from build123d import *

# Parameters (mm, degrees)
BOSS_EXTRUDE1_DEPTH = 10
FILLET1_R           = 0.2
BOSS_EXTRUDE2_START = -0.1
SKETCH2_W           = 1.752559166
SKETCH2_H           = 10
BOSS_EXTRUDE2_DEPTH = 0.6
LPATTERN1_DEPTH     = 10


# Read off the part's stored shape, not the designer's step: LPattern1
with BuildPart() as part:
    # Sketch1 → Boss-Extrude1 (new body)
    with BuildSketch(Plane(origin=(0, 0, 0), x_dir=(1, 0, 0), z_dir=(0, 1, 0))):
        with BuildLine():
            Line((0, 3), (0, 0))
            Line((0, 0), (5, 0))
            Line((5, 0), (5, 3))
            Line((5, 3), (2.982182538, 3))
            ThreePointArc((2.982182538, 3), (3.252447725, 2.695376303), (3.35, 2.3))
            ThreePointArc((3.35, 2.3), (2.104623697, 1.547552275), (2.017817462, 3))
            Line((2.017817462, 3), (0, 3))
        make_face()
    extrude(amount=BOSS_EXTRUDE1_DEPTH)

    # Fillet1
    fillet1_edges = [part.edges().sort_by_distance(p)[0] for p in [
        (2.982182538, 5, -3),
        (2.017817462, 5, -3),
    ]]
    fillet(fillet1_edges, radius=FILLET1_R)

    # Sketch2 → Boss-Extrude2 (add)
    with BuildSketch(Plane(origin=(0, 0, -3), x_dir=(-1, 0, 0), z_dir=(0, 0, -1)).offset(BOSS_EXTRUDE2_START)):
        with Locations((-0.876279583, 5)):
            Rectangle(SKETCH2_W, SKETCH2_H)
        with Locations((-4.123720417, 5)):
            Rectangle(SKETCH2_W, SKETCH2_H)
    extrude(amount=BOSS_EXTRUDE2_DEPTH)

    # LPattern1 outline → LPattern1 (add)
    with BuildSketch(Plane(origin=(0, 0, 0), x_dir=(1, 0, 0), z_dir=(0, 1, 0))):
        with BuildLine():
            ThreePointArc((28.250104185, 2.9), (28.223327872, 2.802728057), (28.247440834, 2.704761905))
            ThreePointArc((28.247440834, 2.704761905), (27.5, 1.45), (26.752559166, 2.704761905))
            ThreePointArc((26.752559166, 2.704761905), (26.776672128, 2.802728057), (26.749895815, 2.9))
            Line((26.749895815, 2.9), (26.752559166, 2.9))
            Line((26.752559166, 2.9), (26.752559166, 3.5))
            Line((26.752559166, 3.5), (23.247440834, 3.5))
            Line((23.247440834, 3.5), (23.247440834, 2.9))
            Line((23.247440834, 2.9), (23.250104185, 2.9))
            ThreePointArc((23.250104185, 2.9), (23.223327872, 2.802728057), (23.247440834, 2.704761905))
            ThreePointArc((23.247440834, 2.704761905), (22.5, 1.45), (21.752559166, 2.704761905))
            ThreePointArc((21.752559166, 2.704761905), (21.776672128, 2.802728057), (21.749895815, 2.9))
            Line((21.749895815, 2.9), (21.752559166, 2.9))
            Line((21.752559166, 2.9), (21.752559166, 3.5))
            Line((21.752559166, 3.5), (18.247440834, 3.5))
            Line((18.247440834, 3.5), (18.247440834, 2.9))
            Line((18.247440834, 2.9), (18.250104185, 2.9))
            ThreePointArc((18.250104185, 2.9), (18.223327872, 2.802728057), (18.247440834, 2.704761905))
            ThreePointArc((18.247440834, 2.704761905), (17.5, 1.45), (16.752559166, 2.704761905))
            ThreePointArc((16.752559166, 2.704761905), (16.776672128, 2.802728057), (16.749895815, 2.9))
            Line((16.749895815, 2.9), (16.752559166, 2.9))
            Line((16.752559166, 2.9), (16.752559166, 3.5))
            Line((16.752559166, 3.5), (13.247440834, 3.5))
            Line((13.247440834, 3.5), (13.247440834, 2.9))
            Line((13.247440834, 2.9), (13.250104185, 2.9))
            ThreePointArc((13.250104185, 2.9), (13.223327872, 2.802728057), (13.247440834, 2.704761905))
            ThreePointArc((13.247440834, 2.704761905), (12.5, 1.45), (11.752559166, 2.704761905))
            ThreePointArc((11.752559166, 2.704761905), (11.776672128, 2.802728057), (11.749895815, 2.9))
            Line((11.749895815, 2.9), (11.752559166, 2.9))
            Line((11.752559166, 2.9), (11.752559166, 3.5))
            Line((11.752559166, 3.5), (8.247440834, 3.5))
            Line((8.247440834, 3.5), (8.247440834, 2.9))
            Line((8.247440834, 2.9), (8.250104185, 2.9))
            ThreePointArc((8.250104185, 2.9), (8.223327872, 2.802728057), (8.247440834, 2.704761905))
            ThreePointArc((8.247440834, 2.704761905), (7.5, 1.45), (6.752559166, 2.704761905))
            ThreePointArc((6.752559166, 2.704761905), (6.776672128, 2.802728057), (6.749895815, 2.9))
            Line((6.749895815, 2.9), (6.752559166, 2.9))
            Line((6.752559166, 2.9), (6.752559166, 3.5))
            Line((6.752559166, 3.5), (5, 3.5))
            Line((5, 3.5), (5, 0))
            Line((5, 0), (30, 0))
            Line((30, 0), (30, 3.5))
            Line((30, 3.5), (28.247440834, 3.5))
            Line((28.247440834, 3.5), (28.247440834, 2.9))
            Line((28.247440834, 2.9), (28.250104185, 2.9))
        make_face()
    extrude(amount=LPATTERN1_DEPTH)


solid = part.part
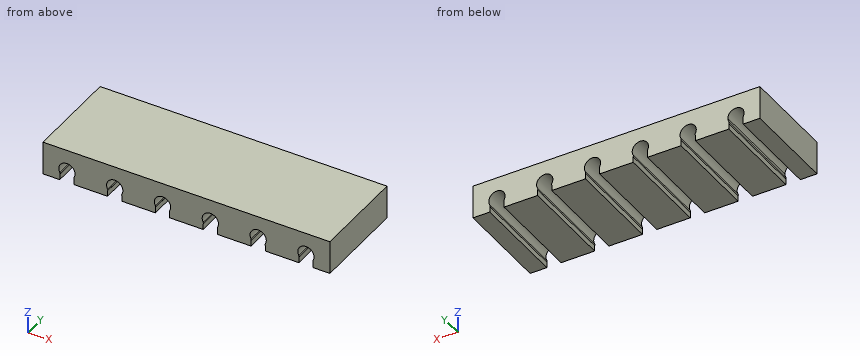
Here's how the part is built. I have some questions about the finished solid (model axes, mm). Give positions to 0.01 mm unless a question says otherwise; leave off trailing zeros. Order: outer loops, then holes, each group sorted by start corner. A loop starts at its lowest first (then second) coordinate and runs counter-clockwise, first axis right, second up. Notation, with made-up numbers: M 67,-30 L 97,-30 A13 cw 97,-10 Z; hole C 67.5,68.25 d7. An arc over 180 degrees is marked long. Answer as a JSON object with one key per item and string values. Group by question number.
1) Please list where this line runs through material, in increasing order: L1, parallel to Z at x = 2.5, y = 5.25. Write a range as [from, to].
2) Suppose I cut it at A-A, the plane z = -1.85. Write out the boundary of the cut face in (x, y), plus the area to 3 significant figures.
3) Suppose I cut it at B-B, the plane x = 27.5. Write out the boundary of the cut face in (y, z), plus the area to 3 significant figures.
Results found:
{
 "1": {"L1": "[-1.45, 0]"},
 "2": {"outline": "M 0,0 L 1.78,0 L 1.78,10 L 0,10 Z; M 3.22,0 L 6.78,0 L 6.78,10 L 3.22,10 Z; M 8.22,0 L 11.78,0 L 11.78,10 L 8.22,10 Z; M 13.22,0 L 16.78,0 L 16.78,10 L 13.22,10 Z; M 18.22,0 L 21.78,0 L 21.78,10 L 18.22,10 Z; M 23.22,0 L 26.78,0 L 26.78,10 L 23.22,10 Z; M 28.22,0 L 30,0 L 30,10 L 28.22,10 Z", "area": "213 mm²"},
 "3": {"outline": "M 0,-1.45 L 10,-1.45 L 10,0 L 0,0 Z", "area": "14.5 mm²"}
}
